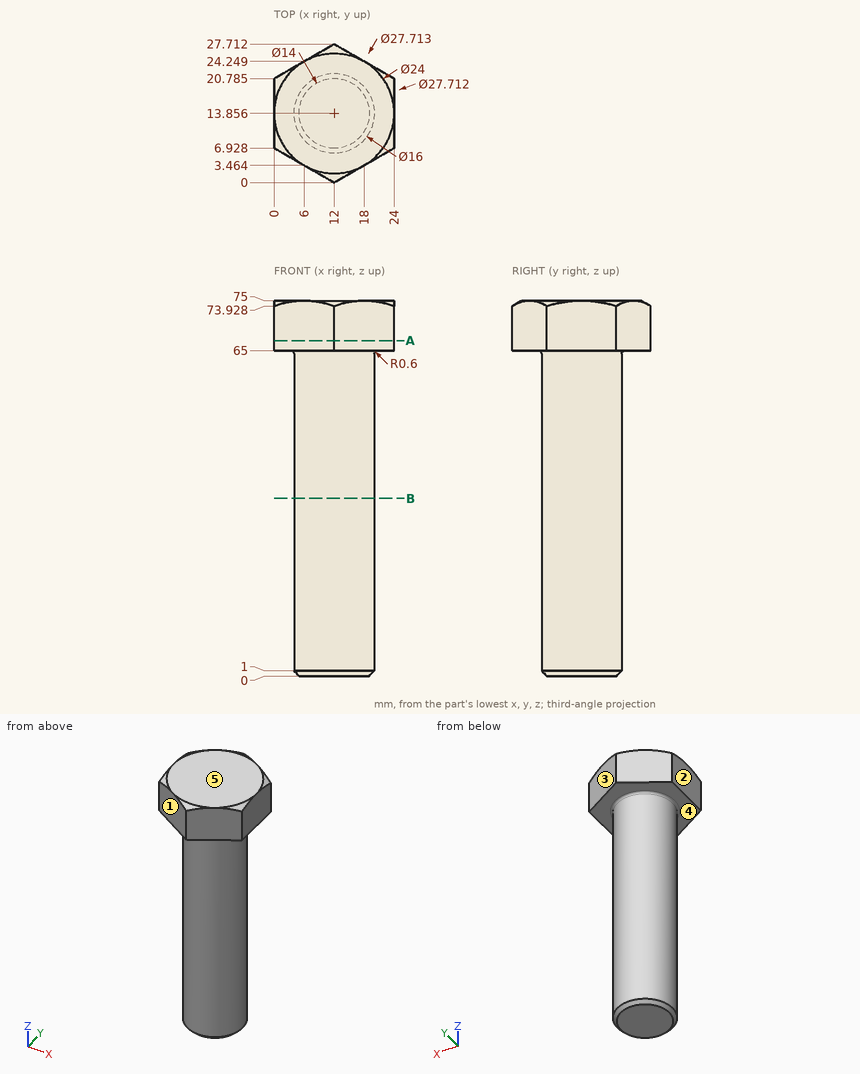
Print and shaded views of the part. All mm, measured from the part's lowest x, y and z. A direction names the side the tool comes from. Give positions to 0.01 mm unless a question says otherwise; leave off trailing zeros. Loops run counter-clockwise (first coordinate to the right, second up) from the corner with the lowest first, then second, coordinate; pieces in that order, holes last. Notation, with made-up numbers: (-39, 37.25) -> (-2, 37.25) arc R13 cw to (-2, 48.25) -> close; hole circle Ø10 at (70.25, 23.5). An arc over 180 degrees is marked (long way). One line per question, with ' | ' between items. Start each with the question number.
1) 3-axis set-ups, long thin cutter, end or side, ignore diameter. For the marked faces 4 and 5: which of +Z, -Z, +X, -X, +Y, -Y reach the whole face in a straight line?
2) Pin check, flat tips, straight feed: pin 1 (4 mm diameter, centred on y = 14, z = 16.5, fed in from -X); pin 2 (1.5 mm diameter, centred on y = 18.5, z = 29.5, fed in from -X); pin 3 (5 mm diameter, centred on y = 8, z = 9.5, fed in from -X). Stop position of each tip, or through.
3) Two-plate mould, pull along Y, no slides. Class the marked faces 1, 2 and 3: released by +Y, released by -Y, zero draft, split by the parting line, or undercut.
4) Cut at A-A (z = 67). Give the cut face in (x, y) (1 decimal).
5) Cut at B-B (z = 35.5). Give the cut face in (x, y).
6) Probe L1, parallel to Y at x = 11.5, z = 46; L2, parallel to Z at x = 16.75, y = 5; L3, parallel to X at y = 10, z = 29.5. List the from-to ranges inside material, lowest first.
Return value:
1) face 4: -Z | face 5: +Z, +X, -X, +Y, -Y
2) pin 1: x = 4 | pin 2: x = 5.01 | pin 3: x = 4.74
3) face 1: released by -Y | face 2: zero draft | face 3: released by +Y
4) outline: (0, 6.9) -> (12, 0) -> (24, 6.9) -> (24, 20.8) -> (12, 27.7) -> (0, 20.8) -> close
5) outline: circle Ø16 at (12, 13.86)
6) L1: 5.87 to 21.84 | L2: 65 to 75 | L3: 4.99 to 19.01
